```python
from build123d import *

# Parameters (mm, degrees)
F0_W     = 96.52
F0_H     = 71.332879
F1_DEPTH = 25.4
F2_R     = 19.327986
F3_DEPTH = 25.4
F5_DEPTH = 71.333879


with BuildPart() as f1:
    # F0 (on Top) → F1 (new body)
    with BuildSketch(Plane.XY):
        with Locations((6.314097, -1.790567)):
            Rectangle(F0_W, F0_H)
    extrude(amount=F1_DEPTH)

    # F2 (on face) → F3 (join)
    with BuildSketch(Plane.XY.offset(25.4)):
        Circle(F2_R)
    extrude(amount=F3_DEPTH)

    # F4 (on face) → F5 (cut, through all)
    with BuildSketch(Plane.XZ.offset(37.457006)):
        Polygon((-20.252686, 51.20115), (54.574097, 25.4), (54.574097, 51.20115), align=None)
    extrude(amount=-F5_DEPTH, mode=Mode.SUBTRACT)


solid = f1.part
```
Geometry: final body of the model. Coordinates: model frame, mm. A direction names the side the tool comes from. Give positions to 0.01 mm unless a question says otherwise; leave off trailing zeros. Order: outer loops, then holes, each group sorted by start corner. A loop starts at its lowest first (then second) coordinate and runs counter-clockwise, first axis right, second up. Notation, with made-up numbers: (-18, 42) -> (41, 42) arc R29 cw to (41, 79) -> close; hole circle Ø6 at (-5.5, 10). An arc over 180 degrees is marked (long way). Write each question's results on one line, items separated by ' | '. Start each with the question number.
1) Section C-C (z = 30). Return loops of the section in (x, y), then the cut area to 3 significant figures.
2) First-contact query: pin 1 (21.5 mm diameter, centred on x = -4.5, y = 15, fed in from +Z); pin 2 (5 mm diameter, centred on y = -17.5, z = 34, fed in from -X); pin 3 (5 mm diameter, centred on x = -21.5, y = -7, fed in from +Z). Flat tips, straight axial feed; report the tip coordinate or a pass-through.
3) Line query: line 1 (Z direction, x = 24, y = -15); line 2 (X direction, y = 3, z = 30.5); line 3 (Z direction, x = -14, y = 3.5). Output: solid intervals per line, ascending. Write a range as from..to.
4) Section B-B (x = 17.5). Return loops of the section in (y, z).
5) Section D-D (y = -13). Return loops of the section in (x, z), then the cut area to 3 significant figures.
6) Set-up query: faces 1 (the flat face through (6, 33.876, 13)), 2 (the flat face through (16, -17, 25.4)). Return all of +Z, -Z, +X, -X, +Y, -Y with unobstructed straight access to the full face (end or side cutting, diameter ignored); none if empty.
7) Section A-A (y = 0). Return loops of the section in (x, z).
Calculated:
1) outline: circle Ø38.66 at (0, 0) | area: 1,170 mm2
2) pin 1: z = 49.36 | pin 2: x = -12.19 | pin 3: z = 25.4
3) line 1: 0..25.4 | line 2: -19.09..19.09 | line 3: 0..49.05
4) outline: (-37.46, 0) -> (33.88, 0) -> (33.88, 25.4) -> (8.2, 25.4) -> (8.2, 38.18) -> (-8.2, 38.18) -> (-8.2, 25.4) -> (-37.46, 25.4) -> close
5) outline: (-41.95, 0) -> (54.57, 0) -> (54.57, 25.4) -> (14.3, 25.4) -> (14.3, 39.29) -> (-14.3, 49.15) -> (-14.3, 25.4) -> (-41.95, 25.4) -> close | area: 2,990 mm2
6) face 1: +Z, -Z, +X, -X, +Y | face 2: +Z
7) outline: (-41.95, 0) -> (54.57, 0) -> (54.57, 25.4) -> (19.33, 25.4) -> (19.33, 37.55) -> (-19.09, 50.8) -> (-19.33, 50.8) -> (-19.33, 25.4) -> (-41.95, 25.4) -> close
